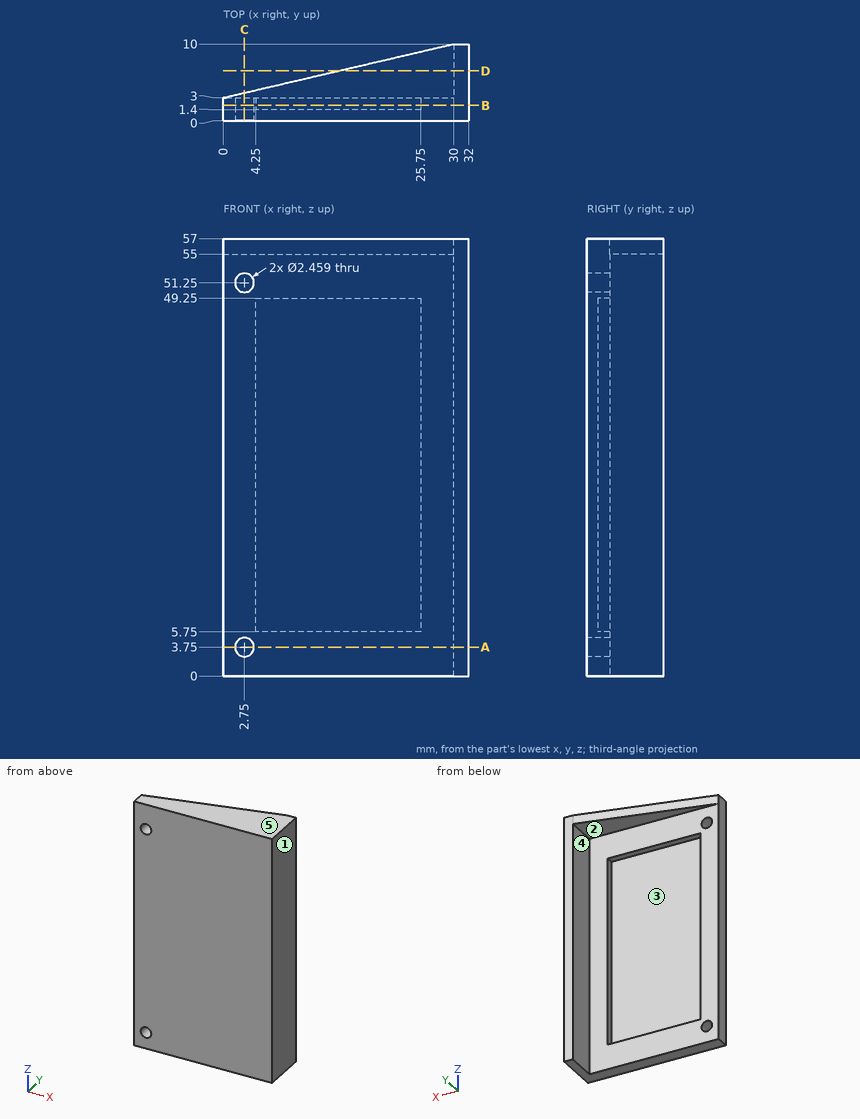
Study the drawing (mm; zero at the part's minimum x, y, z) and answer. A direction names the side the tool comes from. Give positions to 0.01 mm unless a question says otherwise; leave off trailing zeros. Write each loop counter-clockwise with the first axis right and the second up, starting at its lowest first coordinate (ties: lowest second). Pieces come first, ordered by that corner, then holes.
Item 1: Find the intervals of material crossed by line 1 along Z through (x, y) = (2.75, 1.4); line 2 along X through (y, z) = (1.3, 51.25); line 3 along X through (y, z) = (1.5, 11), in increasing order.
Item 2: Which of the six approach directions +Z, -Z, +X, -X, +Y, -Y give full straight-line access (tool end or side, diameter ignored) to the marked faces 1 and 2?
Item 3: Determine the mould class of the marked faces 3, 4 and 5 for opening direction X: released by +X, released by -X, zero draft, split by the parting line, or undercut.
Item 4: Section D-D, the plane y = 6.5 is taken. Write down the section's boundary in (x, z), plus the area to 3 significant figures.
Item 5: Section C-C, the plane x = 2.75 is taken. Write down the section's boundary in (y, z), plus the area to 3 significant figures.
Item 6: Section B-B, the plane y = 2 is taken. Write down the section's boundary in (x, z), plus the area to 3 significant figures.
Item 7: Flat-ended cylindrical pins translate along their axes: P1, Ø1.5, axis at x = 17, z = 47.5, coming from the -Y side; P2, Ø17, axis at x = 17.5, z = 22.5, coming from the +Y side; P3, Ø3.5, axis at y = 7, z = 22.5, coming from the -X side. Find the tip coordinate at first contact, or state that the pin passes through.
Item 8: Section A-A, the plane z = 3.75 is taken. Write down the section's boundary in (x, y), plus the area to 3 significant figures.
Completed:
1. line 1: z = 0 to 2.52, 4.98 to 50.02, 52.48 to 57
1. line 2: x = 0 to 1.52, 3.98 to 32
1. line 3: x = 0 to 4.25, 25.75 to 32
2. face 1: +Z, -Z, +X, +Y, -Y
2. face 2: -Z, -X, +Y
3. face 3: undercut
3. face 4: released by -X
3. face 5: zero draft
4. outline: (15, 55) - (30, 55) - (30, 0) - (32, 0) - (32, 57) - (15, 57) - close
4. area: 144 mm2
5. outline: (0, 0) - (3, 0) - (3, 2.52) - (0, 2.52) - close; (0, 4.98) - (3, 4.98) - (3, 50.02) - (0, 50.02) - close; (0, 52.48) - (3, 52.48) - (3, 55) - (3.64, 55) - (3.64, 57) - (0, 57) - close
5. area: 158 mm2
6. outline: (0, 0) - (32, 0) - (32, 57) - (0, 57) - close; hole circle Ø2.46 at (2.75, 3.75); hole circle Ø2.46 at (2.75, 51.25); hole (4.25, 5.75) - (25.75, 5.75) - (25.75, 49.25) - (4.25, 49.25) - close
6. area: 879 mm2
7. P1: stops at y = 0
7. P2: stops at y = 3
7. P3: stops at x = 30
8. outline: (0, 0) - (1.52, 0) - (1.52, 3) - (0, 3) - close; (3.98, 0) - (32, 0) - (32, 10) - (30, 10) - (30, 3) - (3.98, 3) - close
8. area: 103 mm2
